```python
from build123d import *

# Parameters (mm, degrees)
EXTRUDE_1_DEPTH     = 2
EXTRUDE_2_DEPTH     = 1
EXTRUDE_3_DEPTH     = 1
SKETCH_4_W          = 12
SKETCH_4_H          = 3
CUT_EXTRUDE_1_DEPTH = 3
SKETCH_5_R          = 1.25
CUT_EXTRUDE_2_DEPTH = 3
EXTRUDE_5_REACH     = 5
FILLET_1_R          = 5


with BuildPart() as part:
    # Эскиз1 → Бобышка-Вытянуть1 (new body)
    with BuildSketch(Plane.XY):
        Polygon((8.660254038, 15), (-8.660254038, 15), (-17.320508076, 0), (-8.660254038, -15), (8.660254038, -15), (17.320508076, 0), align=None)
    extrude(amount=EXTRUDE_1_DEPTH)

    # Эскиз2 → Бобышка-Вытянуть2 (add)
    with BuildSketch(Plane.XY.offset(2)):
        Polygon((8.660254038, 15), (-8.660254038, 15), (-17.320508076, 0), (-8.660254038, -15), (8.660254038, -15), (17.320508076, 0), align=None)
        Polygon((7.938566201, 13.75), (-7.938566201, 13.75), (-15.877132403, 0), (-7.938566201, -13.75), (7.938566201, -13.75), (15.877132403, 0), align=None, mode=Mode.SUBTRACT)
    extrude(amount=EXTRUDE_2_DEPTH)

    # Эскиз3 → Бобышка-Вытянуть3 (add)
    with BuildSketch(Plane.XY.offset(2)):
        Polygon((7.361215932, 12.75), (-7.361215932, 12.75), (-14.722431864, 0), (-7.361215932, -12.75), (7.361215932, -12.75), (14.722431864, 0), align=None)
        Polygon((6.639528096, 11.5), (-6.639528096, 11.5), (-13.279056191, 0), (-6.639528096, -11.5), (6.639528096, -11.5), (13.279056191, 0), align=None, mode=Mode.SUBTRACT)
    extrude(amount=EXTRUDE_3_DEPTH)

    # Эскиз4 → Вырез-Вытянуть1 (cut, through all)
    with BuildSketch(Plane.XY.offset(2)):
        with Locations((0, 5.6)):
            Rectangle(SKETCH_4_W, SKETCH_4_H)
    extrude(amount=-CUT_EXTRUDE_1_DEPTH, mode=Mode.SUBTRACT)

    # Эскиз5 → Вырез-Вытянуть2 (cut, through all)
    with BuildSketch(Plane.XY.offset(2)):
        with Locations((-5.484827557, 9.5)):
            Circle(SKETCH_5_R)
        with Locations((5.484827557, 9.5)):
            Circle(SKETCH_5_R)
        with Locations((10.969655115, 0)):
            Circle(SKETCH_5_R)
        with Locations((5.484827557, -9.5)):
            Circle(SKETCH_5_R)
        with Locations((-5.484827557, -9.5)):
            Circle(SKETCH_5_R)
        with Locations((-10.969655115, 0)):
            Circle(SKETCH_5_R)
    extrude(amount=-CUT_EXTRUDE_2_DEPTH, mode=Mode.SUBTRACT)

    # Эскиз7 → Бобышка-Вытянуть5 (add, up to next)
    with BuildSketch(Plane.XY.offset(3), mode=Mode.PRIVATE) as extrude_5_sk1:
        Polygon((-6.75, 11.691342951), (-9.615381057, 13.345671476), (-8.660254038, 15), (-6.75, 15), align=None)
    extrude_5_tool1 = extrude(extrude_5_sk1.sketch, amount=-EXTRUDE_5_REACH, mode=Mode.PRIVATE) - part.part
    add(extrude_5_tool1.solids().sort_by_distance((-7.864315, 13.621393, 3))[0])
    # Эскиз7 → Бобышка-Вытянуть5 (add, up to next)
    with BuildSketch(Plane.XY.offset(3), mode=Mode.PRIVATE) as extrude_5_sk2:
        Polygon((6.75, 11.691342951), (6.75, 15), (8.660254038, 15), (9.615381057, 13.345671476), align=None)
    extrude_5_tool2 = extrude(extrude_5_sk2.sketch, amount=-EXTRUDE_5_REACH, mode=Mode.PRIVATE) - part.part
    add(extrude_5_tool2.solids().sort_by_distance((7.864315, 13.621393, 3))[0])
    # Эскиз7 → Бобышка-Вытянуть5 (add, up to next)
    with BuildSketch(Plane.XY.offset(3), mode=Mode.PRIVATE) as extrude_5_sk3:
        Polygon((13.5, 0), (16.365381057, 1.654328524), (17.320508076, 0), (16.365381057, -1.654328524), align=None)
    extrude_5_tool3 = extrude(extrude_5_sk3.sketch, amount=-EXTRUDE_5_REACH, mode=Mode.PRIVATE) - part.part
    add(extrude_5_tool3.solids().sort_by_distance((15.72863, 0, 3))[0])
    # Эскиз7 → Бобышка-Вытянуть5 (add, up to next)
    with BuildSketch(Plane.XY.offset(3), mode=Mode.PRIVATE) as extrude_5_sk4:
        Polygon((6.75, -11.691342951), (9.615381057, -13.345671476), (8.660254038, -15), (6.75, -15), align=None)
    extrude_5_tool4 = extrude(extrude_5_sk4.sketch, amount=-EXTRUDE_5_REACH, mode=Mode.PRIVATE) - part.part
    add(extrude_5_tool4.solids().sort_by_distance((7.864315, -13.621393, 3))[0])
    # Эскиз7 → Бобышка-Вытянуть5 (add, up to next)
    with BuildSketch(Plane.XY.offset(3), mode=Mode.PRIVATE) as extrude_5_sk5:
        Polygon((-6.75, -11.691342951), (-6.75, -15), (-8.660254038, -15), (-9.615381057, -13.345671476), align=None)
    extrude_5_tool5 = extrude(extrude_5_sk5.sketch, amount=-EXTRUDE_5_REACH, mode=Mode.PRIVATE) - part.part
    add(extrude_5_tool5.solids().sort_by_distance((-7.864315, -13.621393, 3))[0])
    # Эскиз7 → Бобышка-Вытянуть5 (add, up to next)
    with BuildSketch(Plane.XY.offset(3), mode=Mode.PRIVATE) as extrude_5_sk6:
        Polygon((-13.5, 0), (-16.365381057, -1.654328524), (-17.320508076, 0), (-16.365381057, 1.654328524), align=None)
    extrude_5_tool6 = extrude(extrude_5_sk6.sketch, amount=-EXTRUDE_5_REACH, mode=Mode.PRIVATE) - part.part
    add(extrude_5_tool6.solids().sort_by_distance((-15.72863, 0, 3))[0])

    # Скругление1
    fillet_1_edges = [part.edges().sort_by_distance(p)[0] for p in [
        (17.320508076, 0, 1.5),
        (8.660254038, -15, 1.5),
        (-8.660254038, -15, 1.5),
        (-17.320508076, 0, 1.5),
        (-8.660254038, 15, 1.5),
        (8.660254038, 15, 1.5),
    ]]
    fillet(fillet_1_edges, radius=FILLET_1_R)


solid = part.part
```
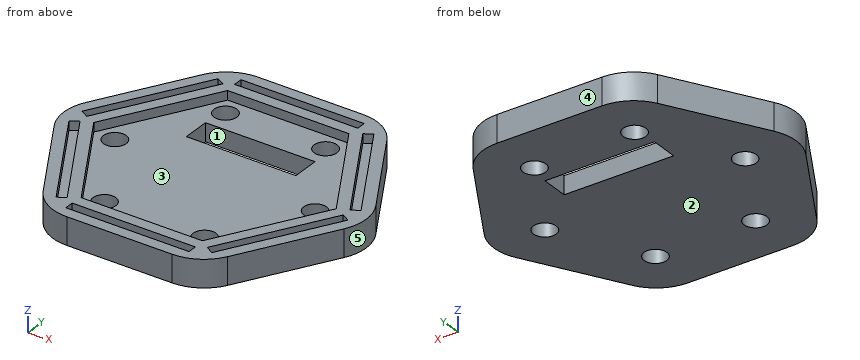
Model file for the job. Use its own axes, mm. Face numbers are marked on the shaded views. A direction names the side the tool comes from. Coordinates: 2 decimals unless noted, no trailing zeros. Order: outer loops, then holes, each group sorted by start corner. A loop starts at its lowest first (then second) coordinate and runs counter-clockwise, first axis right, second up. Notation, with made-up numbers: (43.25, 44.5) -> (75.25, 44.5) arc R14 cw to (75.25, 53.5) -> close; hole circle Ø11 at (59.5, -11.5). An arc over 180 degrees is marked (long way). Return JSON: item names as keys, results as strings.
Item 1: Slice it at C-C (z = 0.8). Write the cut outline in (x, y).
Model answer:
{"outline": "(-15.88, -2.5) -> (-10.1, -12.5) arc R5 ccw to (-5.77, -15) -> (5.77, -15) arc R5 ccw to (10.1, -12.5) -> (15.88, -2.5) arc R5 ccw to (15.88, 2.5) -> (10.1, 12.5) arc R5 ccw to (5.77, 15) -> (-5.77, 15) arc R5 ccw to (-10.1, 12.5) -> (-15.88, 2.5) arc R5 ccw to start; hole circle Ø2.5 at (-10.97, 0); hole circle Ø2.5 at (-5.48, -9.5); hole circle Ø2.5 at (-5.48, 9.5); hole (-6, 4.1) -> (6, 4.1) -> (6, 7.1) -> (-6, 7.1) -> close; hole circle Ø2.5 at (5.48, -9.5); hole circle Ø2.5 at (5.48, 9.5); hole circle Ø2.5 at (10.97, 0)"}
Item 2: Slice it at A-A (x = 3). Write the cut outline in (y, z), then the cut area to 3 significant figures.
Model answer:
{"outline": "(-15, 0) -> (4.1, 0) -> (4.1, 2) -> (-11.5, 2) -> (-11.5, 3) -> (-12.75, 3) -> (-12.75, 2) -> (-13.75, 2) -> (-13.75, 3) -> (-15, 3) -> close; (7.1, 0) -> (15, 0) -> (15, 3) -> (13.75, 3) -> (13.75, 2) -> (12.75, 2) -> (12.75, 3) -> (11.5, 3) -> (11.5, 2) -> (7.1, 2) -> close", "area": "59.0 mm²"}
Item 3: Mould opens along Y. For the marked faces 3, 4 and 5 say: pulls with the +Y half, pulls with the -Y half, needs draft (parallel to the pull), parting line crosses it, or undercut.
Model answer:
{"face 3": "undercut", "face 4": "pulls with the +Y half", "face 5": "parting line crosses it"}
Item 4: Slice it at D-D (y = -9.5). Write the cut outline in (x, z), then the cut area to 3 significant figures.
Model answer:
{"outline": "(-11.84, 0) -> (-6.73, 0) -> (-6.73, 2) -> (-7.79, 2) -> (-7.79, 3) -> (-9.24, 3) -> (-9.24, 2) -> (-10.39, 2) -> (-10.39, 3) -> (-11.84, 3) -> close; (-4.23, 0) -> (4.23, 0) -> (4.23, 2) -> (-4.23, 2) -> close; (6.73, 0) -> (11.84, 0) -> (11.84, 3) -> (10.39, 3) -> (10.39, 2) -> (9.24, 2) -> (9.24, 3) -> (7.79, 3) -> (7.79, 2) -> (6.73, 2) -> close", "area": "43.1 mm²"}
Item 5: 3-axis set-ups, long thin cutter, end or side, ignore diameter. For the marked faces 1 and 2: which of +Z, -Z, +X, -X, +Y, -Y reach the whole face in a straight line?
Model answer:
{"face 1": "+Z, -Z", "face 2": "-Z, +X, -X, +Y, -Y"}
Item 6: Wall check: line 1 along Y through (x, z) = (0.5, 2.55); line 2 along Y through (x, z) = (-3.5, 1.2); line 3 along Y through (x, z) = (15, 2.35). Give the ranges that are in metal, low to high. Write a range as from..to.
Model answer:
{"line 1": "y = -15..-13.75, -12.75..-11.5, 11.5..12.75, 13.75..15", "line 2": "y = -15..4.1, 7.1..15", "line 3": "y = -4.02..-1.52, -0.87..0.87, 1.52..4.02"}
Item 7: Pin check, flat tips, straight feed: P1, Ø1.6, axis at y = 5.5, z = 1.5, coming from the +X side; P2, Ø1, axis at x = -12, z = 0.5, coming from the -Y side; P3, Ø6, axis at x = -11.5, y = 1, coming from the -Z side; P4, Ø0.8, axis at y = 13, z = 2.5, coming from the -X side. Stop position of each tip, or through.
Model answer:
{"P1": "stops at x = 14.61", "P2": "stops at y = -10.08", "P3": "stops at z = 0", "P4": "stops at x = -10.04"}
Item 8: Slice it at B-B (y = 5.5). Write the cut outline in (x, z), then the cut area to 3 significant figures.
Model answer:
{"outline": "(-14.15, 0) -> (-6, 0) -> (-6, 2) -> (-10.1, 2) -> (-10.1, 3) -> (-11.55, 3) -> (-11.55, 2) -> (-12.7, 2) -> (-12.7, 3) -> (-14.15, 3) -> close; (6, 0) -> (14.15, 0) -> (14.15, 3) -> (12.7, 3) -> (12.7, 2) -> (11.55, 2) -> (11.55, 3) -> (10.1, 3) -> (10.1, 2) -> (6, 2) -> close", "area": "38.4 mm²"}
